from build123d import *

# Parameters (mm, degrees)
F0_W     = 86.748682
F0_H     = 56.661889
F1_DEPTH = 70.99464
F2_W     = 12.718076
F2_H     = 13.857008
F3_DEPTH = 53.85619


with BuildPart() as f1:
    # F0 (on Front) → F1 (new body)
    with BuildSketch(Plane.XZ):
        with Locations((1.04402, -28.330944)):
            Rectangle(F0_W, F0_H)
        Polygon((57.705909, 0), (0, 51.346868), (-55.048399, 0), (-42.330321, 0), (44.418361, 0), align=None)
    extrude(amount=-F1_DEPTH)

    # F2 (on Top) → F3 (join)
    with BuildSketch(Plane.XY):
        with Locations((21.544804, 34.737437)):
            Rectangle(F2_W, F2_H)
    extrude(amount=F3_DEPTH)


solid = f1.part
Verification items for the finished model (mm, model axes). A direction names the side the tool comes from. Round coordinates to 2 decimals unless told otherwise and drop trailing zeros. Write each loop counter-clockwise with the first axis right and the second up, starting at its lowest first coordinate (ties: lowest second). Pieces come first, ordered by that corner, then holes.
(1) Section check D-D (y = 35). Enter the section's corners in (x, z).
Returned:
outline: (-55.05, 0) - (-42.33, 0) - (-42.33, -56.66) - (44.42, -56.66) - (44.42, 0) - (57.71, 0) - (27.9, 26.52) - (27.9, 53.86) - (15.19, 53.86) - (15.19, 37.83) - (0, 51.35) - close
(2) Material ranges on line 1 (X direction, y = 10, z = -17); line 2 (Z direction, x = 14, y = 55); line 3 (Z direction, x = 35, y = 27), recorded low to high.
Returned:
line 1: x = -42.33 to 44.42
line 2: z = -56.66 to 38.89
line 3: z = -56.66 to 20.2
(3) Depth check by flat-ended pin: pin 1 Ø8 at (x, y) = (-35.5, 11.5) entering from +Z (3 decimals); pin 2 Ø8 at (x, y) = (-33.5, 24) entering from +Z; pin 3 Ø4 at (x, z) = (19, 44) entering from +Y. Enter the tip coordinate at first touch or a pass-through.
Returned:
pin 1: stops at z = 21.965
pin 2: stops at z = 23.83
pin 3: stops at y = 41.67
(4) Section check A-A (z = 44.5). Enter the section's corners in (x, y), plus the area to 3 significant figures.
Returned:
outline: (-7.34, 0) - (7.69, 0) - (7.69, 70.99) - (-7.34, 70.99) - close; (15.19, 27.81) - (27.9, 27.81) - (27.9, 41.67) - (15.19, 41.67) - close
area: 1,240 mm2
(5) Section check B-B (y = 62.5). Enter the section's corners in (x, z).
Returned:
outline: (-55.05, 0) - (-42.33, 0) - (-42.33, -56.66) - (44.42, -56.66) - (44.42, 0) - (57.71, 0) - (0, 51.35) - close
(6) Access from +Z, -Z, +X, -X, +Y, -Y to the whole of each face (thin tool, end or side, straight path). Record for faces 4 (the flat face through (51, 35, 0)), 5 (the flat face through (-42.33, 35, -29)), 6 (the flat face through (15.186, 35, 46)), 7 (the flat face through (21, 41.666, 43)).
Returned:
face 4: -Z, +X, +Y, -Y
face 5: -Z, -X, +Y, -Y
face 6: +Z, +Y, -Y
face 7: +Z, +X, +Y
(7) Mould release check, pull along Z, two halves, no side actions. Record for faces 1 (the flat face through (-27.14, 35, 26.03)), 2 (the flat face through (27.904, 35, 40)), 3 (the flat face through (0, 35, -56.662)): pulls with the +Z half, pulls with the -Z half, needs draft (parallel to the pull), parting line crosses it, or undercut.
Returned:
face 1: pulls with the +Z half
face 2: needs draft
face 3: pulls with the -Z half
(8) Section check C-C (z = -24). Enter the section's corners in (x, y), plus the area to 3 significant figures.
Returned:
outline: (-42.33, 0) - (44.42, 0) - (44.42, 70.99) - (-42.33, 70.99) - close
area: 6,160 mm2
